```python
from build123d import *

# Parameters (mm, degrees)
F1_DEPTH      = 14
F1_DEPTH_BACK = 14
F3_W          = 6
F3_H          = 1
F4_DEPTH      = 10
F5_R          = 45
F6_DEPTH      = 25
F6_DEPTH_BACK = 25
F7_R          = 2


with BuildPart() as f1:
    # F0 (on Front) → F1 (new body, two sides)
    with BuildSketch(Plane.XZ) as f1_sk:
        with BuildLine():
            Line((-25, 10), (-25, 0))
            Line((-25, 0), (25, 0))
            Line((25, 0), (25, 10))
            ThreePointArc((25, 10), (0, 2.416574), (-25, 10))
        make_face()
    extrude(amount=F1_DEPTH)
    extrude(f1_sk.sketch, amount=-F1_DEPTH_BACK)

    # F3 (on offset) → F4 (join)
    with BuildSketch(Plane.XY.offset(10)):
        with Locations((-15, -13.5)):
            Rectangle(F3_W, F3_H)
        with Locations((-15, 13.5)):
            Rectangle(F3_W, F3_H)
        with Locations((15, -13.5)):
            Rectangle(F3_W, F3_H)
        with Locations((15, 13.5)):
            Rectangle(F3_W, F3_H)
    extrude(amount=-F4_DEPTH)

    # F5 (on Front) → F6 (cut, two sides)
    with BuildSketch(Plane.XZ) as f6_sk:
        with Locations((0, 50)):
            Circle(F5_R)
    extrude(amount=F6_DEPTH, mode=Mode.SUBTRACT)
    extrude(f6_sk.sketch, amount=-F6_DEPTH_BACK, mode=Mode.SUBTRACT)

    # F7
    f7_edges = [f1.edges().sort_by_distance(p)[0] for p in [
        (-25, 14, 5),
        (-25, -14, 5),
        (25, -14, 5),
        (25, 14, 5),
    ]]
    fillet(f7_edges, radius=F7_R)


solid = f1.part
```
Source: CAD feature listing. Evaluate the final solid. Frame: model axes, mm. A direction names the side the tool comes from. Give positions to 0.01 mm unless a question says otherwise; leave off trailing zeros. Order: outer loops, then holes, each group sorted by start corner. A loop starts at its lowest first (then second) coordinate and runs counter-clockwise, first axis right, second up.
(1) Pull-direction query (Y, two-part tool) for faces 4 (the face through (-18, -13.5, 7.5)), 5 (the face through (15, -13, 6)), 6 (the face through (-15, -13, 6)), 7 (the face through (0, -14, 2)); classes: +Y half, -Y half, draft (parallel to the pull), parting line (faces both ways), or undercut.
(2) Material intervals for line 1 along Y through (x, z) = (-14, 4.75); line 2 along Z through (x, y) = (19, -11); line 3 along X through (y, z) = (-3.5, 6), sorted ascending.
(3) Access query for faces 1 (the face through (-18, 13.5, 7.5)), 2 (the face through (-15, 13, 6)), 3 (the face through (25, 0, 5)). Directions: +Z, -Z, +X, -X, +Y, -Y. A direction counts if a zero-diameter tool reaches every point of the face in a straight line with its end or side. Return the directions, or none.
(4) Section query C-C (x = 21). Return the cut outline in (y, z).
(5) Section query A-A (y = -6.75). Return the cut outline in (x, z).
(6) Contact query for flat-ended pins moving along their axis: P1, Ø6, axis at x = 12.5, y = 1.5, coming from the +Z side; P2, Ø10, axis at x = -9, y = -5, coming from the +Z side; P3, Ø0.5, axis at y = -13.5, z = 7.5, coming from the +X side. Output: stop coordinate, or through.
(7) Section query B-B (x = -15). Return the cut outline in (y, z).
Outcome:
1. face 4: draft
1. face 5: undercut
1. face 6: undercut
1. face 7: -Y half
2. line 1: y = -14 to -13, 13 to 14
2. line 2: z = 0 to 6.62
2. line 3: x = -25 to -17.6, 17.6 to 25
3. face 1: +Z, +Y, -Y
3. face 2: +Z
3. face 3: +Z, -Z, +X, +Y, -Y
4. outline: (-14, 0) - (14, 0) - (14, 7.62) - (-14, 7.62) - close
5. outline: (-25, 0) - (25, 0) - (25, 10) arc R45 cw to (-25, 10) - close
6. P1: stops at z = 5.17
6. P2: stops at z = 4.65
6. P3: stops at x = 24.56
7. outline: (-14, 0) - (14, 0) - (14, 7.57) - (13, 7.57) - (13, 4.99) - (-13, 4.99) - (-13, 7.57) - (-14, 7.57) - close
